Could you check a few things on this model? Use its own coordinates, in mm. A direction names the side the tool comes from. Coordinates: 2 decimals unless noted, no trailing zeros. Loops run counter-clockwise (first coordinate to the right, second up) from the corner with the lowest first, then second, coordinate; pieces in that order, holes last.
from build123d import *

# Parameters (mm, degrees)
BOSS_EXTRU_1_DEPTH      = 2
ESQUISSE2_R             = 3
ENL_V_MAT_EXTRU_1_DEPTH = 2
ENL_V_MAT_EXTRU_2_DEPTH = 10
ENL_V_MAT_EXTRU_3_DEPTH = 10
ESQUISSE5_R             = 3
ENL_V_MAT_EXTRU_4_DEPTH = 10


with BuildPart() as part:
    # Esquisse1 → Boss.-Extru.1 (new body)
    with BuildSketch(Plane.XY):
        with BuildLine():
            Line((0, 0), (10, 0))
            Line((10, 0), (10, 18))
            Line((10, 18), (10, 60))
            add(Edge.make_bspline(
                [(10, 60), (-55.226480478, 24.725568105), (0, 42)],
                knots=[0, 0, 0, 1, 1, 1], degree=2))
            Line((0, 42), (0, 0))
        make_face()
    extrude(amount=BOSS_EXTRU_1_DEPTH)

    # Esquisse2 → Enlèv. mat.-Extru.1 (cut)
    with BuildSketch(Plane.XY.offset(2)):
        with Locations((5, 4.288504874)):
            Circle(ESQUISSE2_R)
    extrude(amount=-ENL_V_MAT_EXTRU_1_DEPTH, mode=Mode.SUBTRACT)

    # Esquisse3 → Enlèv. mat.-Extru.2 (cut)
    with BuildSketch(Plane.XY.offset(2)):
        with BuildLine():
            Line((0, 26.586944004), (0, 10.895604928))
            add(Edge.make_bspline(
                [(0, 26.586944004), (6.480930753, 18.900406898), (0, 10.895604928)],
                knots=[0, 0, 0, 1, 1, 1], degree=2))
        make_face()
    extrude(amount=-ENL_V_MAT_EXTRU_2_DEPTH, mode=Mode.SUBTRACT)

    # Esquisse4 → Enlèv. mat.-Extru.3 (cut)
    with BuildSketch(Plane.XY.offset(2)):
        with BuildLine():
            Line((10, 34.129750272), (10, 60))
            add(Edge.make_bspline(
                [(10, 60), (-0.661573878, 54.234228815), (-8.10495368, 49.872428448)],
                knots=[0, 0, 0, 1, 1, 1], degree=2))
            add(Edge.make_bspline(
                [(10, 34.129750272), (9.070365691, 51.175646323), (-8.10495368, 49.872428448)],
                knots=[0, 0, 0, 1, 1, 1], degree=2))
        make_face()
    extrude(amount=-ENL_V_MAT_EXTRU_3_DEPTH, mode=Mode.SUBTRACT)

    # Esquisse5 → Enlèv. mat.-Extru.4 (cut)
    with BuildSketch(Plane(origin=(0, 0, 0), x_dir=(-1, 0, 0), z_dir=(0, 0, -1))):
        with Locations((6.979598084, 46.87242842)):
            Circle(ESQUISSE5_R)
    extrude(amount=-ENL_V_MAT_EXTRU_4_DEPTH, mode=Mode.SUBTRACT)


solid = part.part
(1) Which directions (+Z, -Z, +X, -X, +Y, -Y) give clear straight access to the entire face, cutting with the end or side of a thin tool? Please do faces 4 (the face through (4.35, 1.36, 1.01)), 5 (the face through (0, 6, 1)).
Answers:
face 4: +Z, -Z
face 5: +Z, -Z, -X, -Y
(2) I need wall thicknesses on probe 1 along Y at (x, z) = (-9, 0.75); probe 2 along Y at (x, z) = (-8, 0.6); probe 3 along X at (y, z) = (9, 0.25). Which ranges of each line are inside material? Lowest first, please.
Answers:
probe 1: y = 39.31 to 44.65, 49.09 to 49.35
probe 2: y = 39.59 to 44.05, 49.69 to 49.88
probe 3: x = 0 to 10
(3) Imagine slicing it at B-B, the plane z = 1.5. State how many separate pieces and enclosed holes the cut face has, and give its area (3 significant figures).
Answers:
separate pieces: 1
enclosed holes: 2
area: 556 mm2
(4) Imagine slicing it at A-A, the plane y = 5. Write out the boundary of the cut face in (x, z), and give its area (3 significant figures).
Answers:
outline: (0, 0) - (2.09, 0) - (2.09, 2) - (0, 2) - close; (7.91, 0) - (10, 0) - (10, 2) - (7.91, 2) - close
area: 8.34 mm2
(5) For pin 1 (12 mm diameter, centred on x = -18.5, y = 26.5, fed in from +Z), with a flat end and sliding along its axis, tell me the tip position at first contact or that it passes through.
Answers:
pin 1: passes through
(6) We'd pull the mould along X, two halves only. Please class faces 1 (the face through (5, 0, 1)), 2 (the face through (0, 34, 1)), 3 (the face through (10, 17, 1)): +X half, -X half, draft (parallel to the pull), parting line (faces both ways), or undercut.
Answers:
face 1: draft
face 2: undercut
face 3: +X half
